```python
from build123d import *

# Parameters (mm, degrees)
SKETCH1_R                           = 6.35
SKETCH1_R_2                         = 4.7625
EXTRUDE1_DEPTH                      = 0.508
EXTRUDE2_DEPTH                      = 2.7178
EXTRUDE2_DEPTH_BACK                 = 2.7178
SKETCH3_W                           = 0.611005039
SKETCH3_H                           = 5.4356
EXTRUDE3_DEPTH                      = 0.508
FILLET1_R                           = 1.27
FILLET2_R                           = 1.524
FILLET3_R                           = 2.7178
F_1_32_0_03125_DIAMETER_HOLE1_D     = 2.2098
F_1_32_0_03125_DIAMETER_HOLE1_DEPTH = 6.35


with BuildPart() as part:
    # Sketch1 → Extrude1 (new body)
    with BuildSketch(Plane.XY):
        Circle(SKETCH1_R)
        Circle(SKETCH1_R_2, mode=Mode.SUBTRACT)
    extrude(amount=EXTRUDE1_DEPTH)



with BuildPart() as body_2:
    # Sketch2 → Extrude2 (new, two sides: drawn at the far end of the back side and taken through both)
    with BuildSketch(Plane(origin=(0, 0, 0), x_dir=(1, 0, 0), z_dir=(0, 1, 0)).offset(-EXTRUDE2_DEPTH_BACK)):
        Polygon((-6.35, -0.508), (-6.35, 0), (-6.935979418, 0), (-11.626998738, 7.554015397), (-12.058556542, 7.286019385), (-7.367537222, -0.267996011), (-7.218495515, -0.508), (-6.935979418, -0.508), align=None)
    extrude(amount=EXTRUDE2_DEPTH + EXTRUDE2_DEPTH_BACK)


with BuildPart() as part_1:
    add(part.part)

    add(body_2.part)  # Extrude3 merges body 2
    # Sketch3 → Extrude3 (add)
    with BuildSketch(Plane.XY.offset(0.508)):
        with Locations((-6.044497481, 0)):
            Rectangle(SKETCH3_W, SKETCH3_H)
    extrude(amount=-EXTRUDE3_DEPTH)

    # Fillet1
    fillet1_edges = [part_1.edges().sort_by_distance(p)[0] for p in [
        (-6.935979418, 0, 0),
    ]]
    fillet(fillet1_edges, radius=FILLET1_R)

    # Fillet2
    fillet2_edges = [part_1.edges().sort_by_distance(p)[0] for p in [
        (-7.218495515, 0, 0.508),
    ]]
    fillet(fillet2_edges, radius=FILLET2_R)

    # Fillet3
    fillet3_edges = [part_1.edges().sort_by_distance(p)[0] for p in [
        (-11.84277764, 2.7178, -7.420017391),
        (-11.84277764, -2.7178, -7.420017391),
    ]]
    fillet(fillet3_edges, radius=FILLET3_R - 0.0001)  # a hair under: the kernel refuses the full size

    # 1/32 (0.03125) Diameter Hole1
    with Locations(Plane(origin=(-11.00440601, 0, -5.588505732), x_dir=(-0.527551203197, 0, -0.849523235707), z_dir=(-0.849523235707, 0, 0.527551203197))):
        with Locations((0, 0)):
            Hole(F_1_32_0_03125_DIAMETER_HOLE1_D / 2, depth=F_1_32_0_03125_DIAMETER_HOLE1_DEPTH)


solid = part_1.part
```
Input: part model. Units: mm. Frame: model coordinates. A direction names the side the tool comes from. Give positions to 0.01 mm unless a question says otherwise; leave off trailing zeros. Write each loop counter-clockwise with the first axis right and the second up, starting at its lowest first coordinate (ties: lowest second). Pieces come first, ordered by that corner, then holes. Notation, with made-up numbers: (-25.75, 66) - (-21.75, 66) arc R12 ccw to (-21.75, 80) - close; hole circle Ø1 at (42.5, 5). An arc over 180 degrees is marked (long way). Write item = value, one per line. Start each with the question number.
1. Section query D-D, the plane z = -1.75. Output: boundary loops of the cut face in (x, y), then the cut area to 3 significant figures.
2. Section query C-C, the plane y = 0.5. Count the separate pieces of the cut face and the enclosed holes in it, then the cut area to 3 significant figures.
3. First-contact query: pin 1 Ø4 at (x, y) = (-2, 3.5) entering from -Z; pin 2 Ø1.5 at (y, z) = (-4, -5.5) entering from -X. Flat tips, straight axial feed; report the tip coordinate or a pass-through.
4. Mould query, pull axis X, two halves, no side actions, for faces 4 (the flat face through (-8.4, 2.718, -2)), 5 (the cylindrical face through (-6.839, 0.038, -0.156)), 6 (the cylindrical face through (-3.78, -2.9, 0.25)). Classes: released by +X, released by -X, zero draft, split by the parting line, or undercut.
5. Section query A-A, the plane x = 0. Output: boundary loops of the cut face in (y, z).
6. Access query for faces 1 (the flat face through (-9.405, -0.038, -3.013)), 2 (the flat face through (-8.6, -2.718, -2.1)), 3 (the flat face through (3, -4, 0)). Directions: +Z, -Z, +X, -X, +Y, -Y. A direction counts if a zero-diameter tool reaches every point of the face in a straight line with its end or side. Return the directions, or none.
7. Section query B-B, the plane y = -3.5. Output: boundary loops of the cut face in (x, z), then the cut area to 3 significant figures.
8. Ray query, L1, parallel to Y at x = 0, z = 0.25; L2, parallel to Z at x = -4.75, y = 2; L3, parallel to Z at x = -8.5, y = -2. Return the intervals inside material, ascending.
Check sheet entries:
q1.outline = (-8.62, -2.72) - (-8.02, -2.72) - (-8.02, 2.72) - (-8.62, 2.72) - close
q1.area = 3.25 mm2
q2.separate_pieces = 3
q2.enclosed_holes = 0
q2.area = 5.53 mm2
q3.pin_1 = 0
q3.pin_2 = through
q4.face_4 = zero draft
q4.face_5 = released by +X
q4.face_6 = undercut
q5.outline = (-6.35, 0) - (-4.76, 0) - (-4.76, 0.51) - (-6.35, 0.51) - close; (4.76, 0) - (6.35, 0) - (6.35, 0.51) - (4.76, 0.51) - close
q6.face_1 = +Z, -X, +Y, -Y
q6.face_2 = +Z, -Z, -X, -Y
q6.face_3 = -Z, +X, +Y, -Y
q7.outline = (-5.3, 0) - (-3.23, 0) - (-3.23, 0.51) - (-5.3, 0.51) - close; (3.23, 0) - (5.3, 0) - (5.3, 0.51) - (3.23, 0.51) - close
q7.area = 2.10 mm2
q8.L1 = -6.35 to -4.76, 4.76 to 6.35
q8.L2 = 0 to 0.51
q8.L3 = -2.52 to -1.56
